The model under review builds one solid part; all positions refer to its coordinate system, in mm. Coordinates: 2 decimals unless noted, no trailing zeros. Order: outer loops, then holes, each group sorted by start corner. A loop starts at its lowest first (then second) coordinate and runs counter-clockwise, first axis right, second up. Notation, with made-up numbers: M 29.5,-17 L 63.5,-17 A36 ccw 63.5,19 Z; hole C -20.5,13.25 d6. An arc over 180 degrees is marked long. One line per item, written item: value.
```python
from build123d import *

# Parameters (mm, degrees)
REVOLVE1_ANGLE     = 180
SKETCH3_R          = 26
CUT_EXTRUDE1_DEPTH = 10


with BuildPart() as part:
    # Sketch1 → Revolve1 (revolve)
    with BuildSketch(Plane.XY):
        Polygon((26, 40), (61, 0), (65.013813376, -0.015786716), (30, 40), align=None)
    revolve(axis=Axis((0, 40, 0), (0, -1, 0)), revolution_arc=REVOLVE1_ANGLE)

    # Sketch3 → Cut-Extrude1 (cut)
    with BuildSketch(Plane(origin=(0, 32.212389381, 36.814159292), x_dir=(1, 0, 0), z_dir=(0, 0.6585046078685183, 0.7525766947068778))):
        with Locations((0, -20.352106134)):
            Circle(SKETCH3_R)
    extrude(amount=-CUT_EXTRUDE1_DEPTH, mode=Mode.SUBTRACT)


solid = part.part
```
(1) Mouldability with a two-part tool opening along X and no side actions: class faces 1 (the flat face through (-0.1, 40, 26.2)), 2 (the cylindrical face through (0.922, 34.926, 31.363)), 3 (the conical face through (0.7, 38.06, 31.69)) as +X half, -X half, draft (parallel to the pull), parting line (faces both ways), or undercut.
Geometry results:
face 1: draft
face 2: undercut
face 3: parting line
(2) We need section A-A, the plane x = 0. State the section outline as (y, z) points (1 decimal).
Geometry results:
outline: M 34.5,30.8 L 40,26 L 40,30 L 36.5,33.1 Z
(3) For L1, parallel to X at y = 11, z = 35.5; L2, parallel to X at y = 15.5, z = 9.5; L3, parallel to Y at x = -33, z = 22.5, list the stretches that pass through material, from the lowest coordinate up.
Geometry results:
L1: x = -42.5 to -37.14, 37.14 to 42.5
L2: x = -50.55 to -46.48, 46.48 to 50.55
L3: y = 24.07 to 28.64
(4) Insertion check: pin 1 Ø2 at (x, z) = (36.5, 10.5) entering from +Y; pin 2 Ø3 at (x, z) = (-41, 9.5) entering from +Y; pin 3 Ø4 at (x, y) = (-6.5, 32.5) entering from -Z. Each pin has a flat end and moves straight along its axis. Give the tip position at first contact, or say it passes through.
Geometry results:
pin 1: stops at y = 32.02
pin 2: stops at y = 27.9
pin 3: stops at z = 30.06
